Can you work these out from the model? Positions are in its coordinate system, mm. Face numbers are marked on the shaded views. A direction names the side the tool comes from. Round coordinates to 2 decimals unless told otherwise and drop trailing zeros. Loops run counter-clockwise (first coordinate to the right, second up) from the corner with the lowest first, then second, coordinate; pieces in that order, holes last. Notation, with made-up numbers: (38, 40) -> (52, 40) arc R12 cw to (52, 56) -> close; hole circle Ø4 at (-9.75, 38.5). An arc over 180 degrees is marked (long way). Write each question's results on one line, items separated by ' | '.
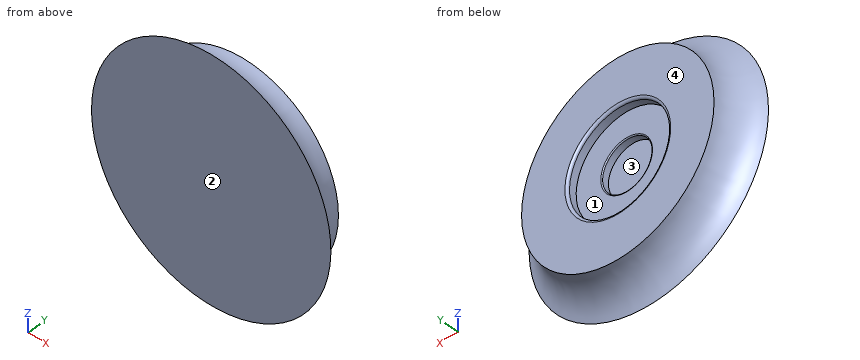
from build123d import *

# Parameters (mm, degrees)
FILLET1_R          = 0.5
SKETCH2_R          = 5.2
CUT_EXTRUDE1_DEPTH = 1.5
FILLET2_R          = 0.2


with BuildPart() as part:
    # Sketch1 → Revolve1 (revolve)
    with BuildSketch(Plane(origin=(0, 0, 0), x_dir=(0, 0, -1), z_dir=(1, 0, 0))):
        with BuildLine():
            Line((0, 0), (-25, 0))
            ThreePointArc((-25, 0), (-21.448462457, 2.728434409), (-20.102542457, 7))
            Line((-20.102542457, 7), (-10.55, 7))
            Line((-10.55, 7), (-10.55, 5))
            Line((-10.55, 5), (0, 5))
            Line((0, 5), (0, 0))
        make_face()
    revolve(axis=Axis((0, 5, 0), (0, -1, 0)))

    # Fillet1
    fillet1_edges = [part.edges().sort_by_distance(p)[0] for p in [
        (0, 7, -10.55),
    ]]
    fillet(fillet1_edges, radius=FILLET1_R)

    # Sketch2 → Cut-Extrude1 (cut)
    with BuildSketch(Plane(origin=(0, 5, 0), x_dir=(1, 0, 0), z_dir=(0, 1, 0))):
        with Locations(Location((0, 0, 0), (0, 0, 270))):
            Circle(SKETCH2_R)
    extrude(amount=-CUT_EXTRUDE1_DEPTH, mode=Mode.SUBTRACT)

    # Fillet2
    fillet2_edges = [part.edges().sort_by_distance(p)[0] for p in [
        (0, 5, -5.2),
    ]]
    fillet(fillet2_edges, radius=FILLET2_R)


solid = part.part
1. Please list where these lines run through material, in increasing order: line 1 (X direction, y = 4.3, z = 0); line 2 (Z direction, x = 4, y = 6.25); line 3 (X direction, y = 6.25, z = 1.5). Write a range as from..to.
Final values:
line 1: -20.61..-5.2, 5.2..20.61 | line 2: -19.74..-9.76, 9.76..19.74 | line 3: -20.08..-10.44, 10.44..20.08
2. We'd pull the mould along Z, two halves only. Please class the marked faces 1 and 2: pulls with the +Z half, pulls with the -Z half, needs draft (parallel to the pull), parting line crosses it, or undercut.
Final values:
face 1: undercut | face 2: needs draft
3. If we section it at B-B (z = 0): List the corners of the cut face in (x, y) for me, then the cut area to 3 significant figures.
Final values:
outline: (-25, 0) -> (25, 0) arc R7.45 cw to (20.1, 7) -> (11.05, 7) arc R0.5 ccw to (10.55, 6.5) -> (10.55, 5) -> (5.4, 5) arc R0.2 ccw to (5.2, 4.8) -> (5.2, 3.5) -> (-5.2, 3.5) -> (-5.2, 4.8) arc R0.2 ccw to (-5.4, 5) -> (-10.55, 5) -> (-10.55, 6.5) arc R0.5 ccw to (-11.05, 7) -> (-20.1, 7) arc R7.45 cw to start | area: 242 mm2
4. On a 3-axis mill with a long thin cutter (end or side, diameter ignored), from which of +Z, -Z, +X, -X, +Y, -Y can I reach the whole of each face in a straight line? I mean the marked faces 3 and 4. Say none if no direction works.
Final values:
face 3: +Y | face 4: +Z, -Z, +X, -X, +Y
5. Will these pins go through, and if not, where does the flat tip stop? pin 1 (1 mm diameter, centred on y = 1, z = 6, fed in from -X); pin 2 (5 mm diameter, centred on x = 0, z = 0.5, fed in from +Y); pin 3 (1 mm diameter, centred on y = 5.5, z = 10, fed in from -X).
Final values:
pin 1: x = -23.15 | pin 2: y = 3.5 | pin 3: x = -17.92
6. If we section it at A-A (x = 0): List the corners of the cut face in (y, z) for me, then the cut area to 3 significant figures.
Final values:
outline: (0, -25) arc R7.45 cw to (7, -20.1) -> (7, -11.05) arc R0.5 ccw to (6.5, -10.55) -> (5, -10.55) -> (5, -5.4) arc R0.2 ccw to (4.8, -5.2) -> (3.5, -5.2) -> (3.5, 5.2) -> (4.8, 5.2) arc R0.2 ccw to (5, 5.4) -> (5, 10.55) -> (6.5, 10.55) arc R0.5 ccw to (7, 11.05) -> (7, 20.1) arc R7.45 cw to (0, 25) -> close | area: 242 mm2
